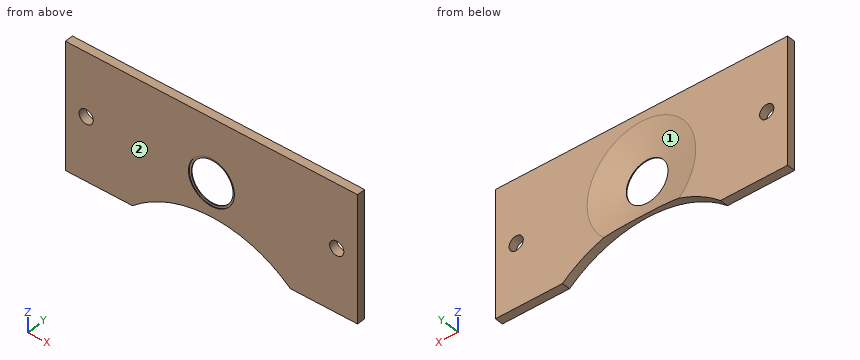
```python
from build123d import *

# Parameters (mm, degrees)
SKETCH1_W            = 70
SKETCH1_H            = 30
SKETCH1_R            = 5
EXTRUDE1_DEPTH       = 2
CHAMFER1_SIZE        = 8
CHAMFER1_SIZE2       = 1.6
SKETCH3_R            = 5.5
CUT_EXTRUDE1_DEPTH   = 0.2
M3_CLEARANCE_HOLE1_D = 3.4
SKETCH7_R            = 28.969188929
CUT_EXTRUDE2_DEPTH   = 3


with BuildPart() as part:
    # Sketch1 → Extrude1 (new body)
    with BuildSketch(Plane(origin=(0, 0, 0), x_dir=(1, 0, 0), z_dir=(0, 1, 0))):
        Rectangle(SKETCH1_W, SKETCH1_H)
        Circle(SKETCH1_R, mode=Mode.SUBTRACT)
    extrude(amount=EXTRUDE1_DEPTH)

    # Chamfer1
    chamfer1_edges = [part.edges().sort_by_distance(p)[0] for p in [
        (-5, 2, 0),
    ]]
    chamfer1_side = [part.faces().sort_by_distance(p)[0] for p in [
        (0, 2, -14.238422689),
    ]]
    chamfer(chamfer1_edges, length=CHAMFER1_SIZE, length2=CHAMFER1_SIZE2, reference=chamfer1_side[0])

    # Sketch3 → Cut-Extrude1 (cut)
    with BuildSketch(Plane.XZ):
        Circle(SKETCH3_R)
    extrude(amount=-CUT_EXTRUDE1_DEPTH, mode=Mode.SUBTRACT)

    # M3 Clearance Hole1 (through all)
    with Locations(Plane(origin=(0, 2, 0), x_dir=(-1, 0, 0), z_dir=(0, 1, 0))):
        with Locations((-30, 0), (30, 0)):
            Hole(M3_CLEARANCE_HOLE1_D / 2)

    # Sketch7 → Cut-Extrude2 (cut, through all)
    with BuildSketch(Plane(origin=(0, 2, 0), x_dir=(-1, 0, 0), z_dir=(0, 1, 0))):
        with Locations((0, -36.93290324)):
            Circle(SKETCH7_R)
    extrude(amount=-CUT_EXTRUDE2_DEPTH, mode=Mode.SUBTRACT)


solid = part.part
```
Check sheet for the modelled part. Datum: model origin and axes. Units: mm. Face numbers are marked on the shaded views. Round coordinates to 2 decimals unless told otherwise and drop trailing zeros. Loops run counter-clockwise (first coordinate to the right, second up) from the corner with the lowest first, then second, coordinate; pieces in that order, holes last. Notation, with made-up numbers: M 43.5,59 L 59.5,59 A18 ccw 59.5,82 Z; hole C 77,11 d5. An arc over 180 degrees is marked long. Answer as a JSON object with one key per item and string values.
1. Scan lines: line 1 (Z direction, x = -30, y = 1.2); line 2 (Z direction, x = 0, y = 0.1); line 3 (X direction, y = 1.85, z = -12.5). Record each from-to range of solid material in increasing order.
Reply:
{"line 1": "z = -15 to -1.7, 1.7 to 15", "line 2": "z = -7.96 to -5.5, 5.5 to 15", "line 3": "x = -35 to -15.56, 15.56 to 35"}
2. Section check C-C (y = 1.5). Record the boundary of the cut face in (x, z).
Reply:
{"outline": "M -35,-15 L -18.93,-15 A28.97 cw -6.03,-8.6 A10.5 cw long 6.03,-8.6 A28.97 cw 18.93,-15 L 35,-15 L 35,15 L -35,15 Z; hole C -30,0 d3.4; hole C 30,0 d3.4"}
3. Section check D-D (x = 0). Record the boundary of the cut face in (y, z), plus the area to 3 significant figures.
Reply:
{"outline": "M 0,-7.96 L 0.99,-7.96 L 0.4,-5 L 0.2,-5 L 0.2,-5.5 L 0,-5.5 Z; M 0,5.5 L 0.2,5.5 L 0.2,5 L 0.4,5 L 2,13 L 2,15 L 0,15 Z", "area": "15.5 mm²"}
4. Section check A-A (z = 0). Record the boundary of the cut face in (x, y).
Reply:
{"outline": "M -35,0 L -31.7,0 L -31.7,2 L -35,2 Z; M -28.3,0 L -5.5,0 L -5.5,0.2 L -5,0.2 L -5,0.4 L -13,2 L -28.3,2 Z; M 5,0.2 L 5.5,0.2 L 5.5,0 L 28.3,0 L 28.3,2 L 13,2 L 5,0.4 Z; M 31.7,0 L 35,0 L 35,2 L 31.7,2 Z"}
5. Gauge pin test, flat ends, axial feed: P1, Ø2, axis at x = -0.5, z = 3, coming from the -Y side; P2, Ø4, axis at x = -30, z = 0, coming from the +Y side. Record the tip position at first contact, or that the pin passes through.
Reply:
{"P1": "passes through", "P2": "stops at y = 2"}
6. Section check B-B (x = 30). Record the boundary of the cut face in (y, z), plus the area to 3 significant figures.
Reply:
{"outline": "M 0,-15 L 2,-15 L 2,-1.7 L 0,-1.7 Z; M 0,1.7 L 2,1.7 L 2,15 L 0,15 Z", "area": "53.2 mm²"}
7. Mould release check, pull along X, two halves, no side actions. Record for the marked faces 1 and 2: pulls with the +X half, pulls with the -X half, needs draft (parallel to the pull), parting line crosses it, or undercut.
Reply:
{"face 1": "undercut", "face 2": "needs draft"}
